Job drawing, mm, ordinate dimensions from the low corner. One solid piece. Coordinates: 2 decimals unless noted, no trailing zeros. Order: outer loops, then holes, each group sorted by start corner. A loop starts at its lowest first (then second) coordinate and runs counter-clockwise, first axis right, second up. Notation, with made-up numbers: (-1.5, 41.25) - (18.5, 41.25) arc R15 ccw to (18.5, 61.25) - close; hole circle Ø1 at (43.5, -7). An arc over 180 degrees is marked (long way). Use a Markdown table: item, result. Add a question column.
1) Drop flat-ended pins along their axis: P1, Ø5, axis at x = 15.5, z = 126.5, coming from the -Y side; P2, Ø10, axis at x = 100.5, y = 17.5, coming from the +Z side; P3, Ø2, axis at x = 84, y = 17, coming from the +Z side; P4, Ø0.9, axis at x = 87.5, z = 74.5, coming from the +Y side. Give the stop position or say it passes through.
2) Saw through at A-A on y = 18. List the corners of the cut face in (x, z).
3) Wall check: L1, parallel to X at y = 47.1, z = 75; L2, parallel to Z at x = 73, y = 5; L3, parallel to X at y = 49.15, z = 75. Give the ranges that are in metal, low to high. Write a range as [from, to].
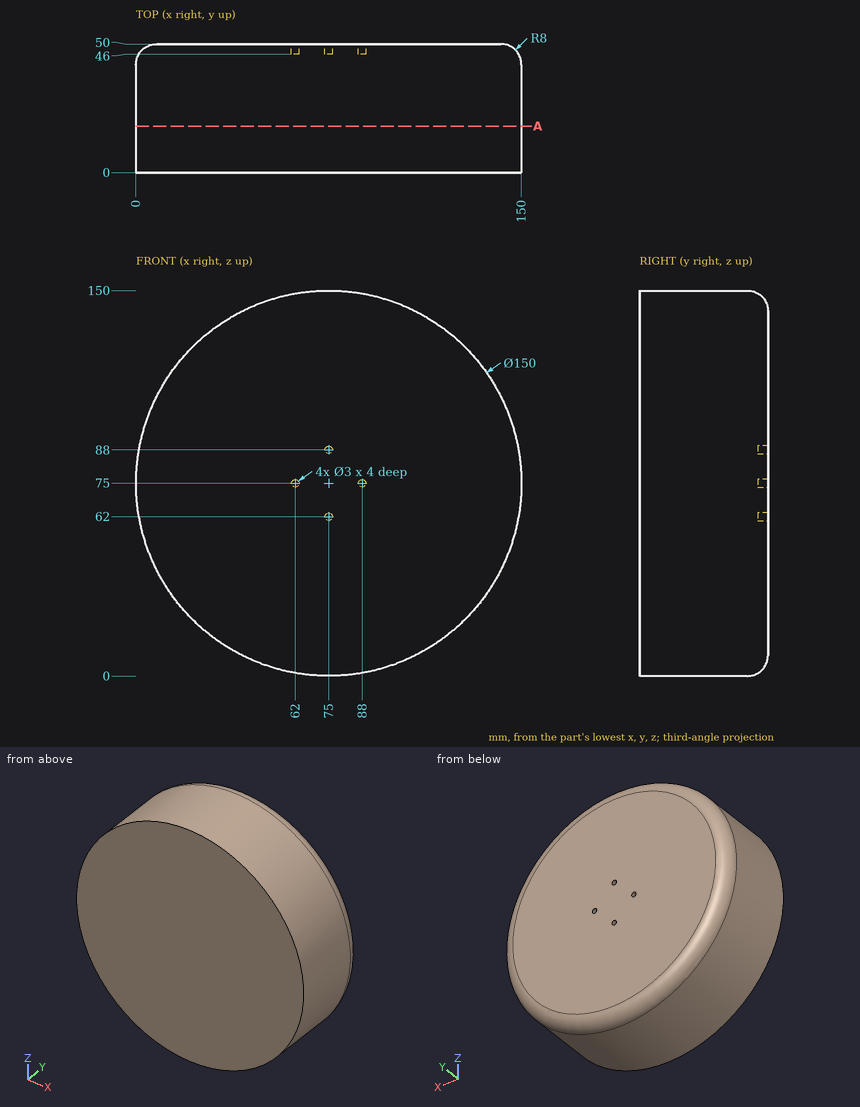
Results are:
| question | item | result |
|---|---|---|
| 1 | P1 | through |
| 1 | P2 | z = 147.14 |
| 1 | P3 | z = 149.57 |
| 1 | P4 | y = 46 |
| 2 | outline | circle Ø150 at (75, 75) |
| 3 | L1 | [1.84, 60.5], [63.5, 86.5], [89.5, 148.16] |
| 3 | L2 | [0.03, 149.97] |
| 3 | L3 | [4.41, 60.5], [63.5, 86.5], [89.5, 145.59] |
